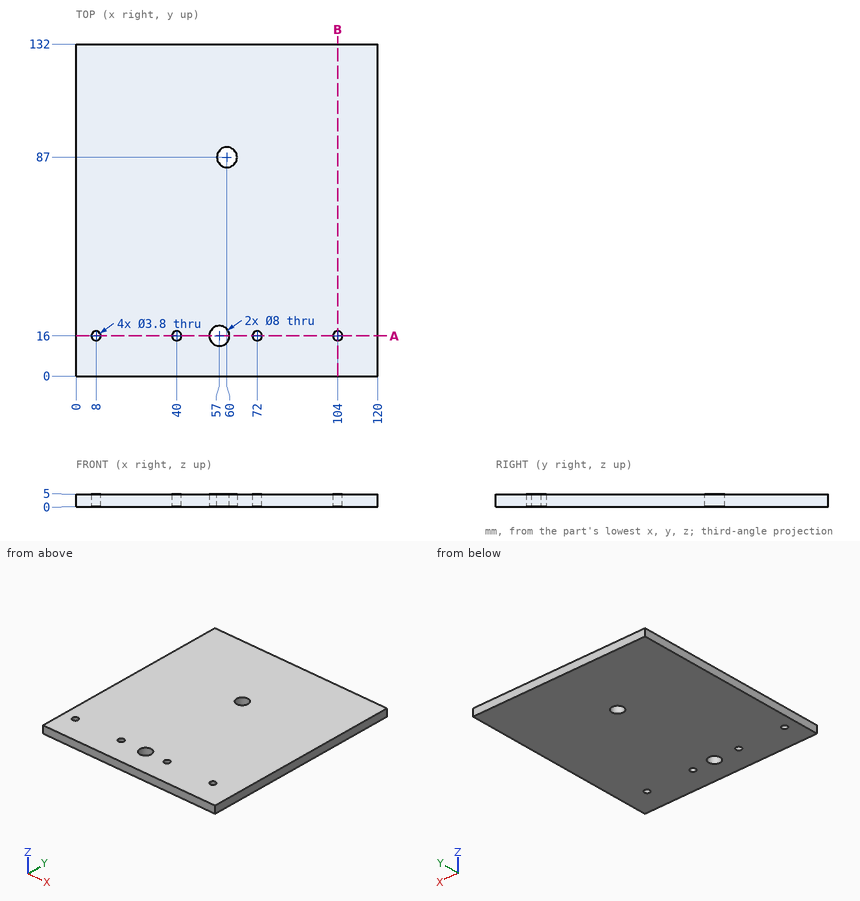
The figure shows three views and two pictorial views of one solid part (mm, origin at its lowest corner). Answer the questions. Coordinates: 2 decimals unless noted, no trailing zeros. Write each loop counter-clockwise with the first axis right and the second up, starting at its lowest first coordinate (ties: lowest second). Pieces come first, ordered by that corner, then holes. Notation, with made-up numbers: (-16.5, -30) -> (-9.5, -30) arc R23 ccw to (-9.5, -8) -> close; hole circle Ø3 at (23.5, 57). An arc over 180 degrees is marked (long way). Return JSON: item names as keys, results as strings.
(1) The part is cut by section A-A on y = 16. Give the vertices of the cut face in (x, z).
Answers below:
{"outline": "(0, 0) -> (6.1, 0) -> (6.1, 5) -> (0, 5) -> close; (9.9, 0) -> (38.1, 0) -> (38.1, 5) -> (9.9, 5) -> close; (41.9, 0) -> (53, 0) -> (53, 5) -> (41.9, 5) -> close; (61, 0) -> (70.1, 0) -> (70.1, 5) -> (61, 5) -> close; (73.9, 0) -> (102.1, 0) -> (102.1, 5) -> (73.9, 5) -> close; (105.9, 0) -> (120, 0) -> (120, 5) -> (105.9, 5) -> close"}
(2) Consider line 1 along Y through (x, z) = (8, 2.4); line 2 along Y through (x, z) = (57, 4.05); line 3 along Y through (x, z) = (54, 0.55). Determine where each line is inside the solid, lowest interval first. Write a range as from..to.
Answers below:
{"line 1": "0..14.1, 17.9..132", "line 2": "0..12, 20..84.35, 89.65..132", "line 3": "0..13.35, 18.65..132"}
(3) The part is cut by section B-B on x = 104. Give the vertices of the cut face in (y, z), then the cut area to 3 significant figures.
Answers below:
{"outline": "(0, 0) -> (14.1, 0) -> (14.1, 5) -> (0, 5) -> close; (17.9, 0) -> (132, 0) -> (132, 5) -> (17.9, 5) -> close", "area": "641 mm^2"}
